Input: part model. Units: mm. Frame: model coordinates. Face numbers are marked on the shaded views. A direction names the side the tool comes from. Coordinates: 2 decimals unless noted, no trailing zeros. Loops run counter-clockwise (first coordinate to the right, second up) from the corner with the lowest first, then second, coordinate; pieces in that order, holes last.
(1) Contact query for flat-ended pins moving along their axis: P1, Ø2.5, axis at y = -2, z = -29.5, coming from the +X side; P2, Ø3, axis at x = -14, z = 2.5, coming from the -Y side; P3, Ø4, axis at x = 4, y = 0.5, coming from the -Z side. Output: stop coordinate, or through.
(2) Section A-A, the plane x = 0. Return loops of the section in (y, z).
(3) Section B-B, the plane z = 2. Return loops of the section in (x, y).
(4) Line query: L1, parallel to X at y = 0.55, z = -37.1; L2, parallel to Z at x = 2, y = 2.5; L3, parallel to Z at x = 5.5, y = 0.75. Output: solid intervals per line, ascending.
(5) Set-up query: the marked faces 5, 6, 7 and 8. Return all of +Z, -Z, +X, -X, +Y, -Y with unobstructed straight access to the full face (end or side cutting, diameter ignored); none if empty.
(6) Mould query, pull axis X, two halves, no side actions, for the marked faces 1, 2, 3 and 4. Classes: released by +X, released by -X, zero draft, split by the parting line, or undercut.
(7) Section D-D, the plane z = -12. Return loops of the section in (x, y), then the cut area to 3 significant figures.
(8) Section C-C, the plane y = 2. Return loops of the section in (x, z), then the cut area to 3 significant figures.
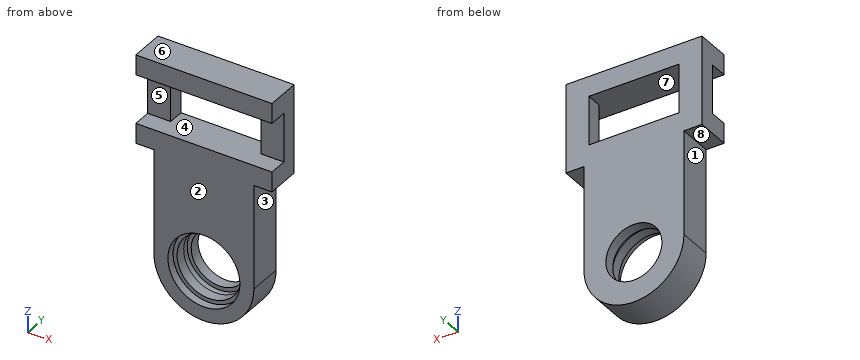
```python
from build123d import *

# Parameters (mm, degrees)
SKETCH1_W           = 34
SKETCH1_H           = 22.2
SKETCH1_W_2         = 22.5
SKETCH1_H_2         = 12.2
BOSS_EXTRUDE1_DEPTH = 4
SKETCH2_R           = 8
BOSS_EXTRUDE3_DEPTH = 4
SKETCH3_R           = 9
SKETCH3_R_2         = 8
BOSS_EXTRUDE4_DEPTH = 2.55
SKETCH4_R           = 9
BOSS_EXTRUDE5_DEPTH = 4.55
SKETCH5_R           = 8
SKETCH5_R_2         = 7
BOSS_EXTRUDE8_DEPTH = 2.65


with BuildPart() as part:
    # Sketch1 → Boss-Extrude1 (new body)
    with BuildSketch(Plane(origin=(0, 0, 0), x_dir=(1, 0, 0), z_dir=(0, 1, 0))):
        Rectangle(SKETCH1_W, SKETCH1_H)
        Rectangle(SKETCH1_W_2, SKETCH1_H_2, mode=Mode.SUBTRACT)
    extrude(amount=BOSS_EXTRUDE1_DEPTH)

    # Sketch2 → Boss-Extrude3 (add, through all)
    with BuildSketch(Plane(origin=(0, 4, 0), x_dir=(1, 0, 0), z_dir=(0, 1, 0))):
        with BuildLine():
            Line((-12.5, 37.1), (-12.5, 11.1))
            Line((-12.5, 11.1), (12.5, 11.1))
            Line((12.5, 11.1), (12.5, 37.1))
            ThreePointArc((12.5, 37.1), (0, 49.6), (-12.5, 37.1))
        make_face()
        with Locations(Location((0, 37.1, 0), (0, 0, 270))):
            Circle(SKETCH2_R, mode=Mode.SUBTRACT)
    extrude(amount=-BOSS_EXTRUDE3_DEPTH)

    # Sketch3 → Boss-Extrude4 (add)
    with BuildSketch(Plane.XZ):
        with Locations(Location((0, -37.1, 0), (0, 0, 270))):
            Circle(SKETCH3_R)
        with Locations(Location((0, -37.1, 0), (0, 0, 90))):
            Circle(SKETCH3_R_2, mode=Mode.SUBTRACT)
    extrude(amount=BOSS_EXTRUDE4_DEPTH)

    # Sketch4 → Boss-Extrude5 (add)
    # profile 1 of 2: a face of its own
    with BuildSketch(Plane.XZ):
        with BuildLine():
            Line((12.5, -11.1), (17, -11.1))
            Line((17, -11.1), (17, -6.1))
            Line((17, -6.1), (11.25, -6.1))
            Line((11.25, -6.1), (-11.25, -6.1))
            Line((-11.25, -6.1), (-17, -6.1))
            Line((-17, -6.1), (-17, -11.1))
            Line((-17, -11.1), (-12.5, -11.1))
            Line((-12.5, -11.1), (-12.5, -37.1))
            ThreePointArc((-12.5, -37.1), (0, -49.6), (12.5, -37.1))
            Line((12.5, -37.1), (12.5, -11.1))
        make_face()
        with Locations(Location((0, -37.1, 0), (0, 0, 270))):
            Circle(SKETCH4_R, mode=Mode.SUBTRACT)
    # profile 2 of 2: a face of its own
    with BuildSketch(Plane.XZ):
        Polygon((11.25, 6.1), (17, 6.1), (17, 11.1), (-17, 11.1), (-17, 6.1), (-11.25, 6.1), align=None)
    extrude(amount=BOSS_EXTRUDE5_DEPTH)

    # Sketch5 → Boss-Extrude8 (add)
    with BuildSketch(Plane(origin=(0, 4, 0), x_dir=(1, 0, 0), z_dir=(0, 1, 0))):
        with Locations(Location((0, 37.1, 0), (0, 0, 270))):
            Circle(SKETCH5_R)
        with Locations(Location((0, 37.1, 0), (0, 0, 270))):
            Circle(SKETCH5_R_2, mode=Mode.SUBTRACT)
    extrude(amount=-BOSS_EXTRUDE8_DEPTH)


solid = part.part
```
Report:
1. P1: stops at x = 12.5
1. P2: stops at y = 0
1. P3: stops at z = -49.44
2. outline: (-4.55, -49.6) - (4, -49.6) - (4, -44.1) - (1.35, -44.1) - (1.35, -45.1) - (-2.55, -45.1) - (-2.55, -46.1) - (-4.55, -46.1) - close; (-4.55, -28.1) - (-2.55, -28.1) - (-2.55, -29.1) - (1.35, -29.1) - (1.35, -30.1) - (4, -30.1) - (4, -6.1) - (-4.55, -6.1) - close; (-4.55, 6.1) - (4, 6.1) - (4, 11.1) - (-4.55, 11.1) - close
3. outline: (-17, 0) - (-11.25, 0) - (-11.25, 4) - (-17, 4) - close; (11.25, 0) - (17, 0) - (17, 4) - (11.25, 4) - close
4. L1: x = -12.5 to -8, 8 to 12.5
4. L2: z = -49.44 to -43.81, -30.39 to -6.1, 6.1 to 11.1
4. L3: z = -48.32 to -42.91, -31.29 to -6.1, 6.1 to 11.1
5. face 5: +X, -X, -Y
5. face 6: +Z, +X, -X, +Y, -Y
5. face 7: -Y
5. face 8: -Z, -X, +Y, -Y
6. face 1: released by -X
6. face 2: zero draft
6. face 3: released by +X
6. face 4: undercut
7. outline: (-12.5, -4.55) - (12.5, -4.55) - (12.5, 4) - (-12.5, 4) - close
7. area: 214 mm2
8. outline: (-17, -11.1) - (-12.5, -11.1) - (-12.5, -37.1) arc R12.5 ccw to (12.5, -37.1) - (12.5, -11.1) - (17, -11.1) - (17, 11.1) - (-17, 11.1) - close; hole (-11.25, -6.1) - (11.25, -6.1) - (11.25, 6.1) - (-11.25, 6.1) - close; hole circle Ø14 at (0, -37.1)
8. area: 1,220 mm2
